from build123d import *

# Parameters (mm, degrees)
BOSS_EXTRU_1_DEPTH      = 10
BOSS_EXTRU_1_DEPTH_BACK = 20
ESQUISSE1_R             = 1
ESQUISSE1_W             = 10
ESQUISSE1_H             = 80
ENL_V_START             = -10
ESQUISSE3_W             = 100
ESQUISSE3_H             = 43
ENL_V_MAT_EXTRU_1_DEPTH = 10


with BuildPart() as part:
    # Esquisse1 → Boss.-Extru.1 (new, two sides: drawn at the far end of the back side and taken through both)
    with BuildSketch(Plane.XY.offset(-20).offset(-BOSS_EXTRU_1_DEPTH_BACK)):
        Polygon((-36.141434162, 52.535821702), (-136.141434162, 52.535821702), (-136.141434162, 19.535821702), (-121.141434162, 19.535821702), (-121.141434162, -100.464178298), (-136.141434162, -100.464178298), (-136.141434162, -133.464178298), (-36.141434162, -133.464178298), (-36.141434162, -100.464178298), (-51.141434162, -100.464178298), (-51.141434162, 19.535821702), (-36.141434162, 19.535821702), align=None)
        with Locations((-111.141434162, -100.464178298)):
            Circle(ESQUISSE1_R, mode=Mode.SUBTRACT)
        with Locations((-61.141434162, -100.464178298)):
            Circle(ESQUISSE1_R, mode=Mode.SUBTRACT)
        with Locations((-61.141434162, 19.535821702)):
            Circle(ESQUISSE1_R, mode=Mode.SUBTRACT)
        with Locations((-111.141434162, 19.535821702)):
            Circle(ESQUISSE1_R, mode=Mode.SUBTRACT)
        with Locations((-126.141434162, 29.535821702)):
            Circle(ESQUISSE1_R, mode=Mode.SUBTRACT)
        with Locations((-126.141434162, 42.535821702)):
            Circle(ESQUISSE1_R, mode=Mode.SUBTRACT)
        with Locations((-96.141434162, 29.535821702)):
            Circle(ESQUISSE1_R, mode=Mode.SUBTRACT)
        with Locations((-96.141434162, 42.535821702)):
            Circle(ESQUISSE1_R, mode=Mode.SUBTRACT)
        with Locations((-76.141434162, 29.535821702)):
            Circle(ESQUISSE1_R, mode=Mode.SUBTRACT)
        with Locations((-76.141434162, 42.535821702)):
            Circle(ESQUISSE1_R, mode=Mode.SUBTRACT)
        with Locations((-46.141434162, 29.535821702)):
            Circle(ESQUISSE1_R, mode=Mode.SUBTRACT)
        with Locations((-46.141434162, 42.535821702)):
            Circle(ESQUISSE1_R, mode=Mode.SUBTRACT)
        with Locations((-66.141434162, -40.464178298)):
            Rectangle(ESQUISSE1_W, ESQUISSE1_H, mode=Mode.SUBTRACT)
        with Locations((-106.141434162, -40.464178298)):
            Rectangle(ESQUISSE1_W, ESQUISSE1_H, mode=Mode.SUBTRACT)
        with Locations((-86.141434162, -40.464178298)):
            Rectangle(ESQUISSE1_W, ESQUISSE1_H, mode=Mode.SUBTRACT)
        with Locations((-46.141434162, -110.464178298)):
            Circle(ESQUISSE1_R, mode=Mode.SUBTRACT)
        with Locations((-46.141434162, -123.464178298)):
            Circle(ESQUISSE1_R, mode=Mode.SUBTRACT)
        with Locations((-76.141434162, -110.464178298)):
            Circle(ESQUISSE1_R, mode=Mode.SUBTRACT)
        with Locations((-126.141434162, -123.464178298)):
            Circle(ESQUISSE1_R, mode=Mode.SUBTRACT)
        with Locations((-126.141434162, -110.464178298)):
            Circle(ESQUISSE1_R, mode=Mode.SUBTRACT)
        with Locations((-96.141434162, -123.464178298)):
            Circle(ESQUISSE1_R, mode=Mode.SUBTRACT)
        with Locations((-96.141434162, -110.464178298)):
            Circle(ESQUISSE1_R, mode=Mode.SUBTRACT)
        with Locations((-76.141434162, -123.464178298)):
            Circle(ESQUISSE1_R, mode=Mode.SUBTRACT)
    extrude(amount=BOSS_EXTRU_1_DEPTH + BOSS_EXTRU_1_DEPTH_BACK)

    # Esquisse3 → Enlèv. mat.-Extru.1 (cut)
    with BuildSketch(Plane(origin=(0, 0, -40), x_dir=(-1, 0, 0), z_dir=(0, 0, -1)).offset(ENL_V_START)):
        with Locations((86.141434162, -111.964178298)):
            Rectangle(ESQUISSE3_W, ESQUISSE3_H)
        with Locations((86.141434162, 31.035821702)):
            Rectangle(ESQUISSE3_W, ESQUISSE3_H)
    extrude(amount=-ENL_V_MAT_EXTRU_1_DEPTH, mode=Mode.SUBTRACT)


solid = part.part
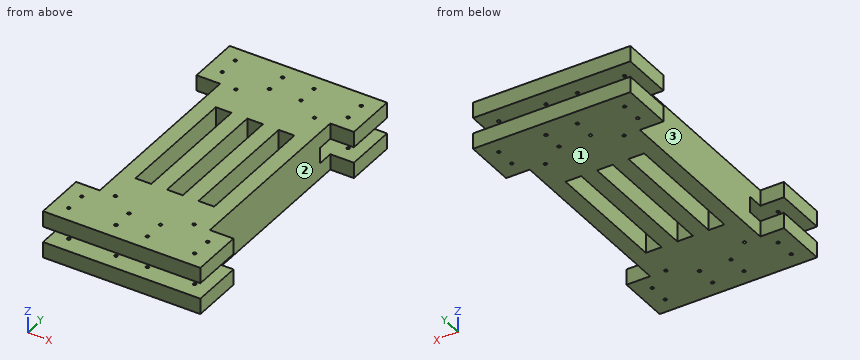
Read the model definition and answer for the solid it produces. Units are mm, in the model's axes. Face numbers are marked on the shaded views. A direction names the side the tool comes from. Round coordinates to 2 decimals unless told otherwise and drop trailing zeros. Loops run counter-clockwise (first coordinate to the right, second up) from the corner with the lowest first, then second, coordinate; pieces in that order, holes last.
Q1. Section B-B on y = 36.5 is taken. Write down the section's boundary in (x, z), and give its area (3 significant figures).
Q2. This flat-tipped pin is pushed along its axis until it touches: pin 1 (4 mm diameter, centred on y = -40, z = -14.5, fed in from -X). Where does it stop, or does it pass through?
Q3. Section C-C on x = -58 is taken. Write down the section's boundary in (y, z), and give its area (3 significant figures).
Q4. Consider probe 1 along X at (y, z) = (-100.5, -12.5); probe 2 along X at (y, z) = (-65, -25); probe 3 along Y at (x, z) = (-104, -31). Determine where each line is inside the solid, lowest interval first.
Q5. Section A-A on z = -24.25 is taken. Write down the section's boundary in (x, y).
Q6. Which of the six approach directions +Z, -Z, +X, -X, +Y, -Y give full straight-line access (tool end or side, diameter ignored) to the marked faces 1, 2 and 3?
Q7. Section D-D on y = -25 is taken. Write down the section's boundary in (x, z), and give its area (3 significant figures).
Output:
1. outline: (-136.14, -40) - (-36.14, -40) - (-36.14, -30) - (-136.14, -30) - close; (-136.14, -20) - (-36.14, -20) - (-36.14, -10) - (-136.14, -10) - close
1. area: 2,000 mm2
2. pin 1: stops at x = -121.14
3. outline: (-133.46, -40) - (52.54, -40) - (52.54, -30) - (9.54, -30) - (9.54, -20) - (52.54, -20) - (52.54, -10) - (-133.46, -10) - (-133.46, -20) - (-90.46, -20) - (-90.46, -30) - (-133.46, -30) - close
3. area: 4,720 mm2
4. probe 1: x = -136.14 to -112.14, -110.14 to -62.14, -60.14 to -36.14
4. probe 2: x = -121.14 to -111.14, -101.14 to -91.14, -81.14 to -71.14, -61.14 to -51.14
4. probe 3: y = -133.46 to -80.46, -0.46 to 52.54
5. outline: (-121.14, -90.46) - (-51.14, -90.46) - (-51.14, 9.54) - (-121.14, 9.54) - close; hole (-111.14, -80.46) - (-101.14, -80.46) - (-101.14, -0.46) - (-111.14, -0.46) - close; hole (-91.14, -80.46) - (-81.14, -80.46) - (-81.14, -0.46) - (-91.14, -0.46) - close; hole (-71.14, -80.46) - (-61.14, -80.46) - (-61.14, -0.46) - (-71.14, -0.46) - close
6. face 1: -Z, +X, -X, +Y, -Y
6. face 2: +Z, -Z, +X
6. face 3: +Z, -Z, -X
7. outline: (-121.14, -40) - (-111.14, -40) - (-111.14, -10) - (-121.14, -10) - close; (-101.14, -40) - (-91.14, -40) - (-91.14, -10) - (-101.14, -10) - close; (-81.14, -40) - (-71.14, -40) - (-71.14, -10) - (-81.14, -10) - close; (-61.14, -40) - (-51.14, -40) - (-51.14, -10) - (-61.14, -10) - close
7. area: 1,200 mm2
